```python
from build123d import *

# Parameters (mm, degrees)
F0_W      = 200
F0_H      = 300
F1_DEPTH  = 1.5
F2_W      = 20
F2_H      = 300
F3_DEPTH  = 200
F4_W      = 24.0114152431
F4_H      = 300
F5_DEPTH  = 200
F6_W      = 199.5166987181
F6_H      = 301.0709583759
F7_DEPTH  = 1.5
F9_R      = 32.6244324659
F10_DEPTH = 1.5
F11_W     = 200
F11_H     = 201.5
F12_DEPTH = 1.5
F13_W     = 199.7538208961
F13_H     = 200.2487033606
F14_DEPTH = 1.5


with BuildPart() as f1:
    # F0 (on Front) → F1 (new body)
    with BuildSketch(Plane.XZ):
        with Locations((100, 150)):
            Rectangle(F0_W, F0_H)
    extrude(amount=F1_DEPTH)

    # F2 (on Front) → F3 (join)
    with BuildSketch(Plane.XZ):
        with Locations((10, 150)):
            Rectangle(F2_W, F2_H)
    extrude(amount=F3_DEPTH)

    # F4 (on face) → F5 (join)
    with BuildSketch(Plane.XZ.offset(1.5)):
        with Locations((187.9942923784, 150)):
            Rectangle(F4_W, F4_H)
    extrude(amount=F5_DEPTH)

    # F6 (on face) → F7 (join)
    with BuildSketch(Plane.XZ.offset(200)):
        with Locations((99.758349359, 150.535479188)):
            Rectangle(F6_W, F6_H)
    extrude(amount=F7_DEPTH)

    # F9 (on face) → F10 (cut)
    with BuildSketch(Plane(origin=(0, 0, 0), x_dir=(-1, 0, 0), z_dir=(0, 1, 0))):
        with Locations((-98.5869541764, 82.1533799171)):
            Circle(F9_R)
    extrude(amount=-F10_DEPTH, mode=Mode.SUBTRACT)

    # F11 (on face) → F12 (join)
    with BuildSketch(Plane(origin=(0, 0, 0), x_dir=(1, 0, 0), z_dir=(0, 0, -1))):
        with Locations((100, 100.75)):
            Rectangle(F11_W, F11_H)
    extrude(amount=F12_DEPTH)

    # F13 (on face) → F14 (join)
    with BuildSketch(Plane.XY.offset(300)):
        with Locations((99.8769104481, -100.1243516803)):
            Rectangle(F13_W, F13_H)
    extrude(amount=F14_DEPTH)


solid = f1.part
```
CAD build for the part. Positions are in the model's coordinates, mm. A direction names the side the tool comes from. Give positions to 0.01 mm unless a question says otherwise; leave off trailing zeros. Order: outer loops, then holes, each group sorted by start corner. A loop starts at its lowest first (then second) coordinate and runs counter-clockwise, first axis right, second up.
(1) Saw through at A-A, the plane x = 171.5. Give the cut face in (y, z), then the cut area to 3 significant figures.
(2) Saw through at C-C, the plane z = 152.5. Give the cut face in (x, y).
(3) Saw through at D-D, the plane x = 127. Give the cut face in (y, z), then the cut area to 3 significant figures.
(4) Tool access for faces 5 (the flat face through (99, 0, 148)), 6 (the cylindrical face through (105.659, -0.74, 50.305)), 7 (the flat face through (175.989, -99, 148)): list every direction of +Z, -Z, +X, -X, +Y, -Y with a clear straight run to the whole face (end or side of a thin tool).
(5) Saw through at B-B, the plane y = -150. Give the cut face in (x, z), then the cut area to 3 significant figures.
(6) Flat gauge pins, fed straight in: pin 1 (0.6 mm diameter, centred on x = 106.5, y = -201, fed in from +Z); pin 2 (0.5 mm diameter, centred on y = -201, z = 300.5, fed in from +X). Where does each tip first touch, or does it go through?
(7) Drill centre lines: L1, parallel to X at y = -164, z = 244; L2, parallel to Y at x = 45, z = 35.5; L3, parallel to Z at x = 131.5, y = -140. Where is each one in solid material? Low to high.
(8) Mould opens along X. For faces 1 (the flat face through (200, -99, 151)), 2 (the flat face through (97, -1.5, 152)), 3 (the flat face through (99, -102, -1.5)), 4 (the flat face through (20, -99, 148)) say: released by +X, released by -X, zero draft, split by the parting line, or undercut.
Results found:
1. outline: (-201.5, -1.5) - (0, -1.5) - (0, 301.5) - (-200.25, 301.5) - (-200.25, 301.07) - (-201.5, 301.07) - close; hole (-200, 0) - (-1.5, 0) - (-1.5, 300) - (-200, 300) - close
1. area: 1,500 mm2
2. outline: (0, -201.5) - (200, -201.5) - (200, 0) - (0, 0) - close; hole (20, -200) - (175.99, -200) - (175.99, -1.5) - (20, -1.5) - close
3. outline: (-201.5, -1.5) - (0, -1.5) - (0, 66.12) - (-1.5, 66.12) - (-1.5, 0) - (-200, 0) - (-200, 300) - (-1.5, 300) - (-1.5, 98.19) - (0, 98.19) - (0, 301.5) - (-200.25, 301.5) - (-200.25, 301.07) - (-201.5, 301.07) - close
3. area: 1,460 mm2
4. face 5: +Z, -Z, +X, -X, +Y
4. face 6: +Y
4. face 7: none
5. outline: (0, -1.5) - (200, -1.5) - (200, 300) - (199.75, 300) - (199.75, 301.5) - (0, 301.5) - close; hole (20, 0) - (175.99, 0) - (175.99, 300) - (20, 300) - close
5. area: 13,800 mm2
6. pin 1: stops at z = 301.07
6. pin 2: stops at x = 199.52
7. L1: x = 0 to 20, 175.99 to 200
7. L2: y = -201.5 to -200, -1.5 to 0
7. L3: z = -1.5 to 0, 300 to 301.5
8. face 1: released by +X
8. face 2: undercut
8. face 3: zero draft
8. face 4: undercut
